```python
from build123d import *

# Parameters (mm, degrees)
SKETCH_1_W          = 89.974599949
SKETCH_1_H          = 53.974599949
EXTRUDE_1_DEPTH     = 16
SHELL_1_T           = -5
SKETCH_2_W          = 11
SKETCH_2_H          = 43.974599949
CUT_EXTRUDE_1_DEPTH = 90.974599949
SKETCH_3_W          = 18.148336296
SKETCH_3_H          = 11
CUT_EXTRUDE_2_DEPTH = 54.974599949
SKETCH_4_R          = 1.524003048
CUT_EXTRUDE_3_DEPTH = 17


with BuildPart() as part:
    # 草图1 → 凸台-拉伸1 (new body)
    with BuildSketch(Plane.XY):
        with Locations((-75.588712629, -507.770940429)):
            Rectangle(SKETCH_1_W, SKETCH_1_H)
    extrude(amount=-EXTRUDE_1_DEPTH)

    # 抽壳1
    shell_1_openings = [part.faces().sort_by_distance(p)[0] for p in [
        (-75.588712629, -507.770940429, 0),
    ]]
    offset(amount=SHELL_1_T, openings=shell_1_openings, kind=Kind.INTERSECTION)

    # 草图2 → 切除-拉伸1 (cut, through all)
    with BuildSketch(Plane.ZY.offset(120.576012603)):
        with Locations((-5.5, -507.770940429)):
            Rectangle(SKETCH_2_W, SKETCH_2_H)
    extrude(amount=-CUT_EXTRUDE_1_DEPTH, mode=Mode.SUBTRACT)

    # 草图3 → 切除-拉伸2 (cut, through all)
    with BuildSketch(Plane.XZ.offset(534.758240403)):
        with Locations((-111.501844455, -5.5)):
            Rectangle(SKETCH_3_W, SKETCH_3_H)
    extrude(amount=-CUT_EXTRUDE_2_DEPTH, mode=Mode.SUBTRACT)

    # 草图4 → 切除-拉伸3 (cut, through all)
    with BuildSketch(Plane.XY):
        with Locations((-105.092649637, -483.310945509)):
            Circle(SKETCH_4_R)
        with Locations((-54.038547528, -526.999032885)):
            Circle(SKETCH_4_R)
        with Locations((-54.038547528, -498.296975481)):
            Circle(SKETCH_4_R)
    extrude(amount=-CUT_EXTRUDE_3_DEPTH, mode=Mode.SUBTRACT)


solid = part.part
```
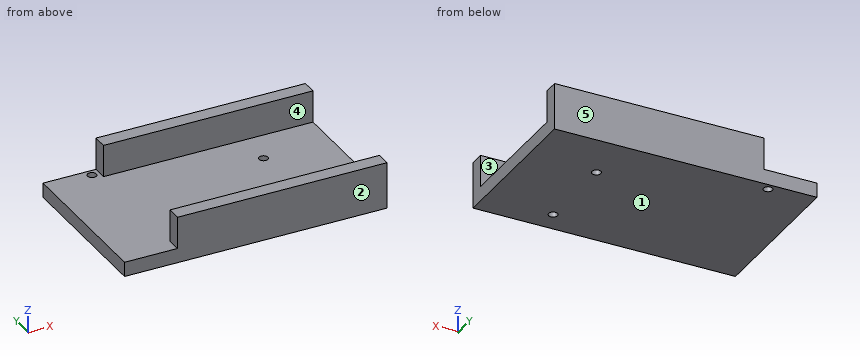
Build history of the part. All positions in model axes, mm. Face numbers are marked on the shaded views. A direction names the side the tool comes from. Round coordinates to 2 decimals unless told otherwise and drop trailing zeros. Loops run counter-clockwise (first coordinate to the right, second up) from the corner with the lowest first, then second, coordinate; pieces in that order, holes last.
Item 1: Pin check, flat tips, straight feed: P1, Ø16, axis at x = -69.5, y = -510, coming from the +Z side; P2, Ø5, axis at y = -509.5, z = -9, coming from the +X side; P3, Ø5.5, axis at y = -482.5, z = -3.5, coming from the -X side. Stop position of each tip, or through.
Item 2: Saw through at C-C (y = -505.5). List the corners of the cut face in (x, z), then the cut area to 3 significant figures.
Item 3: Saw through at B-B (x = -85.5). List the corners of the cut face in (y, z), then the cut area to 3 significant figures.
Item 4: Saw through at A-A (z = -1.5). List the corners of the cut face in (x, y).
Item 5: Drill centre lines: line 1 along Y through (x, z) = (-61, -10.25); line 2 along Z through (x, y) = (-38, -512); line 3 along X through (y, z) = (-531, -3.5). Where is each one in solid material? Low to high.
Item 6: Two-plate mould, pull along Y, no slides. Class the marked faces 1, 2 and 3: released by +Y, released by -Y, zero draft, split by the parting line, or undercut.
Item 7: Saw through at D-D (x = -112). List the corners of the cut face in (y, z), then the cut area to 3 significant figures.
Item 8: Which spindle directions (+Z, -Z, +X, -X, +Y, -Y) get a long thin tool onto all of the face, cutting with end or side? Do the marked faces 4 and 5. Say none if no direction does.
Worked answers:
1. P1: stops at z = -11
1. P2: stops at x = -30.6
1. P3: stops at x = -102.43
2. outline: (-120.58, -16) - (-30.6, -16) - (-30.6, -11) - (-120.58, -11) - close
2. area: 450 mm2
3. outline: (-534.76, -16) - (-480.78, -16) - (-480.78, 0) - (-485.78, 0) - (-485.78, -11) - (-529.76, -11) - (-529.76, 0) - (-534.76, 0) - close
3. area: 380 mm2
4. outline: (-102.43, -534.76) - (-30.6, -534.76) - (-30.6, -529.76) - (-102.43, -529.76) - close; (-102.43, -485.78) - (-30.6, -485.78) - (-30.6, -480.78) - (-102.43, -480.78) - close
5. line 1: y = -534.76 to -529.76, -485.78 to -480.78
5. line 2: z = -16 to -11
5. line 3: x = -102.43 to -30.6
6. face 1: zero draft
6. face 2: released by -Y
6. face 3: undercut
7. outline: (-534.76, -16) - (-480.78, -16) - (-480.78, -11) - (-534.76, -11) - close
7. area: 270 mm2
8. face 4: +Z, +X, -X
8. face 5: +Z, -Z, +X, -X, +Y
